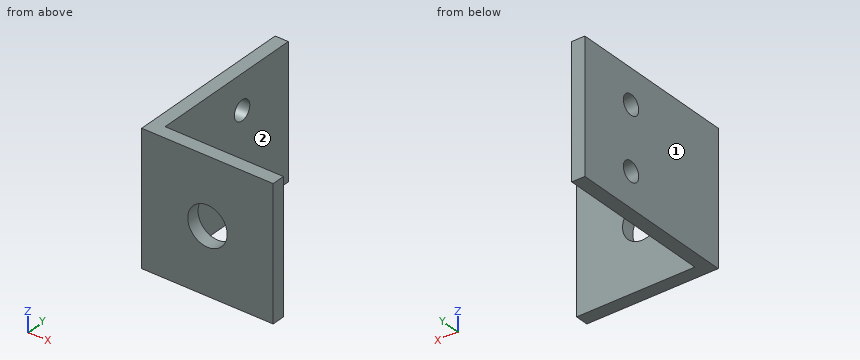
Autodesk Inventor part; units mm, degrees
ref_plane "YZ Plane" through (0, 0, 0) normal (1, 0, 0) x (0, 1, 0)
ref_plane "XZ Plane" through (0, 0, 0) normal (0, 1, 0) x (-1, 0, 0)
ref_plane "XY Plane" through (0, 0, 0) normal (0, 0, 1) x (1, 0, 0)
sketch "Sketch9" plane through (0, 0, 0) normal (0, 0, 1) x (1, 0, 0)
  line L0 (0, 0) -> (20, 0)
  line L1 (20, 0) -> (20, 26)
  line L2 (2, 26) -> (0, 26)
  line L3 (0, 26) -> (0, 0)
  line L4 (2, 26) -> (2, 2)
  line L5 (2, 2) -> (20, 2)
  line L6 (20, 2) -> (20, 26)
  dimension "d35" = 20
  dimension "d36" = 26
  dimension "d37" = 2
  dimension "d38" = 2
extrude "Extrusion9" add sketch "Sketch9" against normal blind 20
sketch "Sketch10" plane through (0, 0, 0) normal (0, -1, 0) x (1, 0, 0)
  line L0 (0, 0) -> (20, 0)
  line L1 (10, 0) -> (10, -20)
  line L2 (20, -20) -> (0, -20)
  circle A0 centre (10, -10) radius 3
  dimension "d41" = 6
extrude "Extrusion10" cut sketch "Sketch10" against normal through all
sketch "Sketch11" plane through (0, 0, 0) normal (-1, 0, 0) x (0, 0, 1)
  line L0 (0, 26) -> (0, 0)
  line L1 (0, 26) -> (0, 17)
  circle A0 centre (-5.25, 17) radius 1.5
  circle A1 centre (-14.75, 17) radius 1.5
  dimension "d44" = 9
  dimension "d45" = 3
  dimension "d46" = 3
  dimension "d47" = 9.5
  dimension "d48" = 5.25
extrude "Extrusion11" cut sketch "Sketch11" against normal through all
properties part number "LimitSwitch MountV2"
Input: part model. Units: mm. Frame: model coordinates. Face numbers are marked on the shaded views. A direction names the side the tool comes from. Give positions to 0.01 mm unless a question says otherwise; leave off trailing zeros. Write each loop counter-clockwise with the first axis right and the second up, starting at its lowest first coordinate (ties: lowest second). Pieces come first, ordered by that corner, then holes.
Q1. Set-up query: the marked faces 1 and 2. Return all of +Z, -Z, +X, -X, +Y, -Y with unobstructed straight access to the full face (end or side cutting, diameter ignored); none if empty.
Q2. Section B-B, the plane x = 10. Output: boundary loops of the cut face in (y, z).
Q3. Section D-D, the plane z = -10. Output: boundary loops of the cut face in (x, y).
Q4. First-contact query: P1, Ø4, axis at y = 5, z = -5, coming from the +X side; P2, Ø2.5, axis at y = 17, z = -5.25, coming from the +X side; P3, Ø8, axis at x = 17, z = -16, coming from the +Y side. Flat tips, straight axial feed; report the tip coordinate or a pass-through.
Q5. Section C-C, the plane y = 17. Output: boundary loops of the cut face in (x, z), plus the area to 3 significant figures.
Q6. Section A-A, the plane z = -14.75. Output: boundary loops of the cut face in (x, y).
Q7. Material intervals for probe 1 along X at (y, z) = (1.6, -10); probe 2 along Y at (x, z) = (0.7, -5.25); probe 3 along X at (y, z) = (8.5, -16), sorted ascending.
Filled in:
1. face 1: +Z, -Z, -X, +Y, -Y
1. face 2: +Z, -Z, +X, +Y
2. outline: (0, -20) - (2, -20) - (2, -13) - (0, -13) - close; (0, -7) - (2, -7) - (2, 0) - (0, 0) - close
3. outline: (0, 0) - (7, 0) - (7, 2) - (2, 2) - (2, 26) - (0, 26) - close; (13, 0) - (20, 0) - (20, 2) - (13, 2) - close
4. P1: stops at x = 2
4. P2: passes through
4. P3: stops at y = 2
5. outline: (0, -20) - (2, -20) - (2, -16.25) - (0, -16.25) - close; (0, -13.25) - (2, -13.25) - (2, -6.75) - (0, -6.75) - close; (0, -3.75) - (2, -3.75) - (2, 0) - (0, 0) - close
5. area: 28.0 mm2
6. outline: (0, 0) - (20, 0) - (20, 2) - (2, 2) - (2, 15.5) - (0, 15.5) - close; (0, 18.5) - (2, 18.5) - (2, 26) - (0, 26) - close
7. probe 1: x = 0 to 7, 13 to 20
7. probe 2: y = 0 to 15.5, 18.5 to 26
7. probe 3: x = 0 to 2
